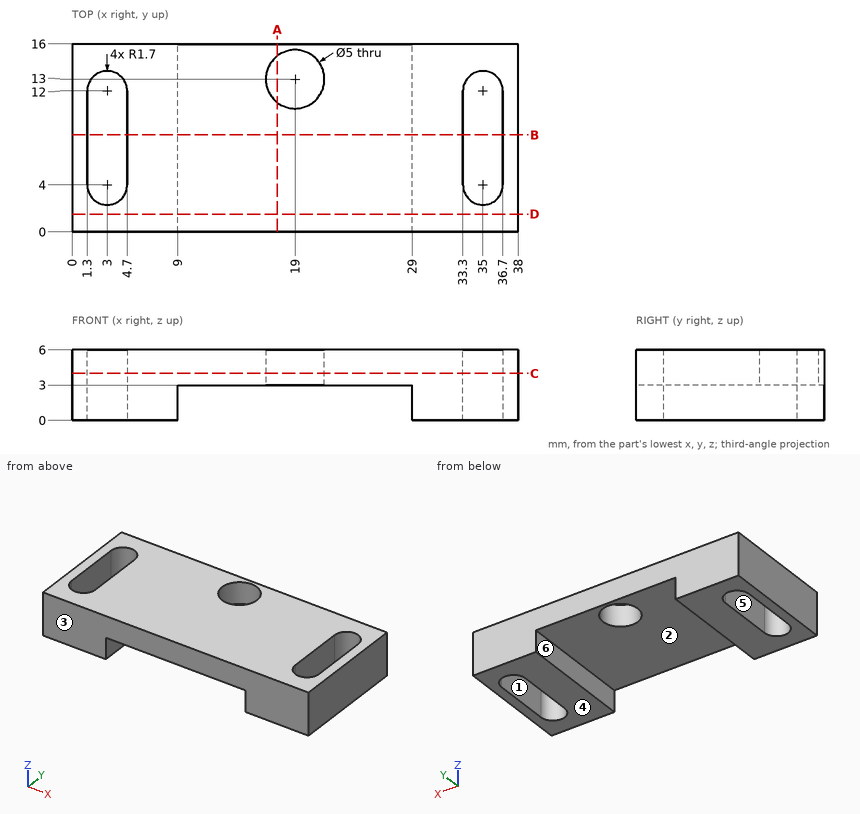
Verification items for this drawing (mm, ordinates from the low corner). A direction names the side the tool comes from. Coordinates: 2 decimals unless noted, no trailing zeros. Write each loop counter-clockwise with the first axis right and the second up, starting at its lowest first coordinate (ties: lowest second). Pieces come first, ordered by that corner, then holes. Notation, with made-up numbers: M 79,-9 L 138,-9 A10 cw 138,-3 Z; hole C -10.5,-5.5 d4. An arc over 180 degrees is marked long. Answer as a JSON object with one key per item and string values. Group by question number.
(1) Release check for a two-part mould opening along Y. For the marked faces 1, 2 and 3 record: +Y half, -Y half, draft (parallel to the pull), parting line (faces both ways), or undercut.
(2) Cross-section at D-D, the plane y = 1.5. Record the cut outline in (x, z).
(3) Cross-section at A-A, the plane x = 17.5. Record the cut outline in (y, z), and give its area (3 significant figures).
(4) Tool access check on the marked faces 4, 5 and 6. Record the directions out of +Z, -Z, +X, -X, +Y, -Y that give a thin tool (end or side, any length) a straight path to the whole face; none if there is none.
(5) Cross-section at C-C, the plane z = 4. Record the cut outline in (x, y).
(6) Cross-section at B-B, the plane y = 8.25. Record the cut outline in (x, z).
(7) Material ranges on line 1 (X direction, y = 8, z = 3.45); line 2 (X direction, y = 9.75, z = 2.45); line 3 (Y direction, x = 19, z = 3.9), recorded low to high.
(8) Gauge pin test, flat end, axial feed: pin 1 (5 mm diameter, centred on x = 16, y = 7, fed in from -Z). Record the tip position at first contact, or that the pin passes through.
Reply:
{
 "1": {"face 1": "undercut", "face 2": "draft", "face 3": "-Y half"},
 "2": {"outline": "M 0,0 L 9,0 L 9,3 L 29,3 L 29,0 L 38,0 L 38,6 L 0,6 Z"},
 "3": {"outline": "M 0,3 L 11,3 L 11,6 L 0,6 Z; M 15,3 L 16,3 L 16,6 L 15,6 Z", "area": "36.0 mm²"},
 "4": {"face 4": "-Z, +X, -X, +Y, -Y", "face 5": "+Z, -Z", "face 6": "-Z, +Y, -Y"},
 "5": {"outline": "M 0,0 L 38,0 L 38,16 L 0,16 Z; hole M 1.3,4 A1.7 ccw 4.7,4 L 4.7,12 A1.7 ccw 1.3,12 Z; hole C 19,13 d5; hole M 33.3,4 A1.7 ccw 36.7,4 L 36.7,12 A1.7 ccw 33.3,12 Z"},
 "6": {"outline": "M 0,0 L 1.3,0 L 1.3,6 L 0,6 Z; M 4.7,0 L 9,0 L 9,3 L 29,3 L 29,0 L 33.3,0 L 33.3,6 L 4.7,6 Z; M 36.7,0 L 38,0 L 38,6 L 36.7,6 Z"},
 "7": {"line 1": "0 to 1.3, 4.7 to 33.3, 36.7 to 38", "line 2": "0 to 1.3, 4.7 to 9, 29 to 33.3, 36.7 to 38", "line 3": "0 to 10.5, 15.5 to 16"},
 "8": {"pin 1": "z = 3"}
}
